Source: CAD feature listing. Evaluate the final solid. Frame: model axes, mm. A direction names the side the tool comes from. Coordinates: 2 decimals unless noted, no trailing zeros. Order: outer loops, then holes, each group sorted by start corner. A loop starts at its lowest first (then second) coordinate and runs counter-clockwise, first axis right, second up. Notation, with made-up numbers: (-9.75, 22) -> (22.25, 22) arc R18 ccw to (22.25, 55) -> close; hole circle Ø11 at (65.5, -15). An arc over 180 degrees is marked (long way). Write item = value, one per line. Start each with the question number.
Item 1: Set-up query: faces 1 (the flat face through (5.866, -76, 14)), 2 (the flat face through (-16.359, -65, 9)), 3 (the flat face through (33.171, 12, 9)), 4 (the flat face through (-44.934, -75, 14)). Return all of +Z, -Z, +X, -X, +Y, -Y with unobstructed straight access to the full face (end or side cutting, diameter ignored); none if empty.
Item 2: Contact query for flat-ended pins moving along their axis: pin 1 (9.5 mm diameter, centred on y = -74.5, z = 10, fed in from -X); pin 2 (2 mm diameter, centred on x = 16, z = 16, fed in from -Y); pin 3 (3 mm diameter, centred on x = -60.5, z = 11, fed in from -Y). Output: stop coordinate, or through.
Item 3: Section query C-C (z = 12.5). Output: boundary loops of the cut face in (x, y) (1 decimal), then the cut area to 3 significant figures.
Item 4: Mould query, pull axis Y, two halves, no side actions, for faces 5 (the cylindrical face through (-21.165, 23.174, 9.392)), 6 (the flat face through (-72.239, 11, 9)), 7 (the flat face through (-5, -84.741, 9)). Classes: released by +Y, released by -Y, zero draft, split by the parting line, or undercut.
Item 5: Section query A-A (y = -65). Output: boundary loops of the cut face in (x, z), then the cut area to 3 significant figures.
Item 6: Section query B-B (x = -37.5). Count the separate pieces of the cut face and the enclosed holes in it, then the cut area to 3 significant figures.
Item 7: Ray query, line 1 along Y through (x, z) = (-23, 8); line 2 along X through (y, z) = (-55, 15); line 3 along Y through (x, z) = (4, 15.5). Return the intervals inside material, ascending. Write a range as [from, to].
Autodesk Inventor part; units mm, degrees
ref_plane "YZ Plane" through (0, 0, 0) normal (1, 0, 0) x (0, 1, 0)
ref_plane "XZ Plane" through (0, 0, 0) normal (0, 1, 0) x (-1, 0, 0)
ref_plane "XY Plane" through (0, 0, 0) normal (0, 0, 1) x (1, 0, 0)
sketch "Sketch1" plane through (0, 0, 0) normal (0, 0, 1) x (1, 0, 0)
  line L0 (-72.2389, 37.814) -> (33.1711, 37.814)
  line L1 (33.1711, 37.814) -> (33.1711, 28.0212)
  line L2 (33.1711, 28.0212) -> (-72.2389, 28.0212)
  line L3 (-72.2389, 28.0212) -> (-72.2389, 37.814)
  circle A0 centre (-19.5339, -14.891) radius 38.1
  circle A1 centre (-19.5339, -14.891) radius 52.705
  line L4 (-72.2389, -14.891) -> (-72.2389, 28.0212)
  line L5 (33.1711, 28.0212) -> (33.1711, -14.891)
  line L6 (-44.9339, -61.0717) -> (-44.9339, -84.741)
  line L7 (-44.9339, -84.741) -> (5.8661, -84.741)
  line L8 (5.8661, -84.741) -> (5.8661, -61.0717)
  line L9 (-22.7089, -52.8585) -> (-22.7089, -84.741)
  line L10 (-16.3589, -84.741) -> (-16.3589, -52.8585)
  point P0 (0, 0)
  dimension "d0" = 105.41
  dimension "d1" = 105.41
  dimension "d2" = 76.2
  dimension "d3" = 52.705
  dimension "d4" = 25.4
  dimension "d5" = 25.4
  dimension "d6" = 69.85
  dimension "d7" = 22.225
  dimension "d8" = 22.225
extrude "Extrusion1" add sketch "Sketch1" along normal blind 19.05 contours L0 A1 L2 L3 | L0 L1 L2 A1 | A1 L2 | A1 L10 A0 L9 L2 | A1 L9 L7 L6 | L8 L7 L10 A1
sketch "Sketch2" plane through (0, 0, 19.05) normal (0, 0, 1) x (1, 0, 0)
  line L0 (-50.1339, 28.0212) -> (-72.2389, 28.0212)
  arc A0 (-50.1339, 28.0212) -> (-44.9339, -61.0717) centre (-19.5339, -14.891) ccw
  arc A1 (5.8661, -61.0717) -> (11.0661, 28.0212) centre (-19.5339, -14.891) ccw
  line L1 (33.1711, 28.0212) -> (11.0661, 28.0212)
  line L2 (33.1711, 37.814) -> (33.1711, 28.0212)
  line L3 (-72.2389, 28.0212) -> (-72.2389, -14.891)
  line L4 (33.1711, 28.0212) -> (33.1711, -14.891)
  point P0 (0, 0)
extrude "Extrusion2" add sketch "Sketch2" against normal blind 19.05
sketch "Sketch3" plane through (5.8661, -84.741, 0) normal (1, 0, 0) x (0, 0, -1)
  point P0 (0, 84.741)
  point P1 (-9.525, 11.8347)
hole "Hole1" at (5.8661, -72.9064, 9.525) direction (-1, 0, 0) diameter 9.525 end through all
properties part number "Router mount"
Computed:
q1.face_1 = +Z, -Z, +X, -Y
q1.face_2 = +Z, -Z, -Y
q1.face_3 = +Z, -Z, +X, +Y, -Y
q1.face_4 = +Z, -Z, -X, -Y
q2.pin_1 = -44.93
q2.pin_2 = -54.71
q2.pin_3 = -49.82
q3.outline = (-72.2, -14.9) arc R52.7 ccw to (-44.9, -61.1) -> (-44.9, -69.2) -> (-22.7, -69.2) -> (-22.7, -52.9) arc R38.1 cw (long way) to (-16.4, -52.9) -> (-16.4, -69.2) -> (5.9, -69.2) -> (5.9, -61.1) arc R52.7 ccw to (33.2, -14.9) -> (33.2, 37.8) -> (-72.2, 37.8) -> close; (-44.9, -84.7) -> (-22.7, -84.7) -> (-22.7, -76.6) -> (-44.9, -76.6) -> close; (-16.4, -84.7) -> (5.9, -84.7) -> (5.9, -76.6) -> (-16.4, -76.6) -> close
q3.area = 5,800 mm^2
q4.face_5 = undercut
q4.face_6 = zero draft
q4.face_7 = released by -Y
q5.outline = (-44.93, 0) -> (-22.71, 0) -> (-22.71, 19.05) -> (-44.93, 19.05) -> close; (-16.36, 0) -> (5.87, 0) -> (5.87, 19.05) -> (-16.36, 19.05) -> close
q5.area = 847 mm^2
q6.separate_pieces = 2
q6.enclosed_holes = 1
q6.area = 983 mm^2
q7.line_1 = [-84.74, -77.42], [-68.39, -52.83], [23.05, 37.81]
q7.line_2 = [-53.73, -22.71], [-16.36, 14.66]
q7.line_3 = [-84.74, -44.85], [15.07, 37.81]
